```python
from build123d import *

# Parameters (mm, degrees)
F1_DEPTH    = 12
F2_DEPTH    = 50
F3_T1_DEPTH = 120.7987304743
F3_T3_DEPTH = 107.0496265693
F4_T1_DEPTH = 64.7830881456
F4_T3_DEPTH = 66.9231117077


# Not quite as in the source:
# - a fillet or chamfer that OpenCascade refuses, or shapes differently, is made with other operations: its cross-section is extruded or revolved along the edge and cut away or added


with BuildPart() as f1:
    # F0 (on Top) → F1 (new body)
    with BuildSketch(Plane.XY):
        with BuildLine():
            ThreePointArc((64.2798563582, -215.6225870974), (32.480131643, -222.643304522), (0, -225))
            Line((0, -225), (0, -250))
            ThreePointArc((0, -250), (36.0890351588, -247.3814494688), (71.4220626202, -239.5806523304))
            Line((71.4220626202, -239.5806523304), (64.2798563582, -215.6225870974))
        make_face()
        with BuildLine():
            ThreePointArc((57.1376500962, -191.6645218643), (28.8712281271, -197.9051595751), (0, -200))
            Line((0, -200), (0, -225))
            ThreePointArc((0, -225), (32.480131643, -222.643304522), (64.2798563582, -215.6225870974))
            Line((64.2798563582, -215.6225870974), (57.1376500962, -191.6645218643))
        make_face()
        with BuildLine():
            ThreePointArc((52.1381057128, -174.8938762012), (26.344995666, -180.5884581123), (0, -182.5))
            Line((0, -182.5), (0, -200))
            ThreePointArc((0, -200), (28.8712281271, -197.9051595751), (57.1376500962, -191.6645218643))
            Line((57.1376500962, -191.6645218643), (52.1381057128, -174.8938762012))
        make_face()
    extrude(amount=F1_DEPTH)

    # F0 (on Top) → F2 (join)
    with BuildSketch(Plane.XY):
        with BuildLine():
            ThreePointArc((57.1376500962, -191.6645218643), (28.8712281271, -197.9051595751), (0, -200))
            Line((0, -200), (0, -225))
            ThreePointArc((0, -225), (32.480131643, -222.643304522), (64.2798563582, -215.6225870974))
            Line((64.2798563582, -215.6225870974), (57.1376500962, -191.6645218643))
        make_face()
    extrude(amount=F2_DEPTH)

    # F3: fillet of radius 20 on 4 edges, made by hand

    # F3_s2 → F3_t1 (cut)
    with BuildSketch(Plane.XY.offset(-54.3993652372)):
        with BuildLine():
            ThreePointArc((21.7391304348, -249.0530268998), (6.4867215062, -243.8729803633), (0, -229.1287847478))
            Line((0, -229.1287847478), (0, -250))
            ThreePointArc((0, -250), (10.8798730474, -249.7631445239), (21.7391304348, -249.0530268998))
        make_face()
        with BuildLine():
            ThreePointArc((50.3184233293, -244.883760739), (63.4552732198, -235.5621710033), (65.4594016494, -219.5792948702))
            Line((65.4594016494, -219.5792948702), (71.4220626202, -239.5806523304))
            ThreePointArc((71.4220626202, -239.5806523304), (60.9279674657, -242.4619202689), (50.3184233293, -244.883760739))
        make_face()
    extrude(amount=F3_T1_DEPTH, mode=Mode.SUBTRACT)

    # F3_s4 → F3_t3 (cut)
    with BuildSketch(Plane.XY.offset(-47.5248132847)):
        with BuildLine():
            ThreePointArc((18.024691358, -181.6077104681), (5.1759288176, -188.0843186765), (0, -201.5099253139))
            Line((0, -201.5099253139), (0, -182.5))
            ThreePointArc((0, -182.5), (9.0233818378, -182.2767911178), (18.024691358, -181.6077104681))
        make_face()
        with BuildLine():
            ThreePointArc((34.609719823, -179.1882175082), (48.7732703354, -181.7241570951), (57.5690180175, -193.111517431))
            Line((57.5690180175, -193.111517431), (52.1381057128, -174.8938762012))
            ThreePointArc((52.1381057128, -174.8938762012), (43.42702673, -177.2578442535), (34.609719823, -179.1882175082))
        make_face()
    extrude(amount=F3_T3_DEPTH, mode=Mode.SUBTRACT)

    # F4: fillet of radius 11 on 4 edges, made by hand

    # F4_s2 → F4_t1 (cut)
    with BuildSketch(Plane.XY.offset(12)):
        with BuildLine():
            ThreePointArc((0, -210.7130750571), (3.0216525247, -203.140362758), (10.4265402844, -199.7280332294))
            Line((10.4265402844, -199.7280332294), (10.3691943128, -198.6295290467))
            ThreePointArc((10.3691943128, -198.6295290467), (5.2147333965, -198.83162866), (0.0567649923, -198.8999918998))
            Line((0.0567649923, -198.8999918998), (-1.0397817327, -199.9169455148))
            ThreePointArc((-1.0397817327, -199.9169455148), (-1.1, -201.5099253139), (-1.1, -210.7130750571))
            Line((-1.1, -210.7130750571), (0, -210.7130750571))
        make_face()
        with BuildLine():
            ThreePointArc((60.1982497665, -201.9311039069), (55.1390969064, -195.5372531202), (47.0679630938, -194.3826300115))
            Line((47.0679630938, -194.3826300115), (46.8090892968, -193.3135255465))
            ThreePointArc((46.8090892968, -193.3135255465), (51.8064632167, -192.0346332539), (56.768991531, -190.6265763228))
            Line((56.768991531, -190.6265763228), (58.1103687488, -191.2878754492))
            ThreePointArc((58.1103687488, -191.2878754492), (58.6231728877, -192.7972603555), (61.2524046367, -201.6168468313))
            Line((61.2524046367, -201.6168468313), (60.1982497665, -201.9311039069))
        make_face()
    extrude(amount=F4_T1_DEPTH, mode=Mode.SUBTRACT)

    # F4_s4 → F4_t3 (cut)
    with BuildSketch(Plane.XY.offset(12)):
        with BuildLine():
            ThreePointArc((0, -213.7171027316), (3.4243688767, -221.6926787663), (11.5654205607, -224.7025612833))
            ThreePointArc((11.5654205607, -224.7025612833), (5.7846223415, -224.9256280293), (0, -225))
            Line((0, -225), (0, -213.7171027316))
        make_face()
        with BuildLine():
            ThreePointArc((61.0564651772, -204.8099315465), (60.0533434239, -213.4314083362), (53.1114776019, -218.6416496163))
            ThreePointArc((53.1114776019, -218.6416496163), (58.7150747837, -217.2039133928), (64.2798563582, -215.6225870974))
            Line((64.2798563582, -215.6225870974), (61.0564651772, -204.8099315465))
        make_face()
    extrude(amount=F4_T3_DEPTH, mode=Mode.SUBTRACT)


solid = f1.part
```
Geometry check sheet. Reference: the model listing, model coordinates, mm. A direction names the side the tool comes from. Round coordinates to 2 decimals unless told otherwise and drop trailing zeros. Loops run counter-clockwise (first coordinate to the right, second up) from the corner with the lowest first, then second, coordinate; pieces in that order, holes last. Notation, with made-up numbers: (-4, -25.5) -> (23, -25.5) arc R9 ccw to (23, -20.5) -> close; hole circle Ø1 at (-11.75, 80.25). An arc over 180 degrees is marked (long way). Use a Markdown table: item, result.
(1) Set-up check for faces 1 (the flat face through (30, -209, 50)), 2 (the cylindrical face through (60.115, -213.323, 30.734)), 3 (the cylindrical face through (2.94, -203.23, 30.73)), 4 (the cylindrical face through (32.189, -222.686, 30.734)): record each of +Z, -Z, +X, -X, +Y, -Y from which the full face is reachable in a straight line by a thin tool's end or side.
Calculated:
| item | result |
|---|---|
| face 1 | +Z, +X, -X, +Y, -Y |
| face 2 | +Z, +X |
| face 3 | +Z, -X, +Y |
| face 4 | +Z, +X, -Y |
(2) Sectioned sample at C-C (y = -207.5). Enter the section's corners in (x, z), then the cut area to 3 significant figures.
Calculated:
| item | result |
|---|---|
| outline | (0, 0) -> (61.86, 0) -> (61.86, 12) -> (61.51, 12) -> (61.51, 50) -> (0.48, 50) -> (0.48, 12) -> (0, 12) -> close |
| area | 3,060 mm² |
(3) Sectioned sample at B-B (x = 38.5). Enter the section's corners in (y, z).
Calculated:
| item | result |
|---|---|
| outline | (-247.02, 0) -> (-178.83, 0) -> (-178.83, 12) -> (-196.26, 12) -> (-196.26, 50) -> (-221.68, 50) -> (-221.68, 12) -> (-247.02, 12) -> close |
(4) Sectioned sample at A-A (z = 9.5). Enter the section's corners in (x, y), then the cut area to 3 significant figures.
Calculated:
| item | result |
|---|---|
| outline | (0, -229.13) arc R20 ccw to (21.74, -249.05) arc R250 ccw to (50.32, -244.88) arc R20 ccw to (65.46, -219.58) -> (57.57, -193.11) arc R20 ccw to (34.61, -179.19) arc R182.5 cw to (18.02, -181.61) arc R20 ccw to (0, -201.51) -> close |
| area | 3,890 mm² |
(5) Go/stop test with flat-tipped pins: P1, Ø1.5, axis at x = 32, z = 25.5, coming from the +Y side; P2, Ø2, axis at x = 51, y = -238.5, coming from the +Z side; P3, Ø5, axis at x = 28.5, z = 30, coming from the -Y side. Record where each tip stops, or that it passes through.
Calculated:
| item | result |
|---|---|
| P1 | y = -197.3 |
| P2 | z = 12 |
| P3 | y = -223.49 |
(6) Sectioned sample at D-D (y = -233). Enter the section's corners in (x, z).
Calculated:
| item | result |
|---|---|
| outline | (0.38, 0) -> (64.75, 0) -> (64.75, 12) -> (0.38, 12) -> close |
(7) Scan lines: probe 1 along Z at (x, y) = (26.5, -197.5); probe 2 along Y at (x, z) = (17.5, 8); probe 3 along Y at (x, z) = (34, 15). Record each from-to range of solid material in increasing order.
Calculated:
| item | result |
|---|---|
| probe 1 | 0 to 12 |
| probe 2 | -248.97 to -181.67 |
| probe 3 | -222.42 to -197.09 |
